Part model, mm, in its own coordinate system. Face numbers are marked on the shaded views. A direction names the side the tool comes from. Give positions to 0.01 mm unless a question says otherwise; leave off trailing zeros. Write each loop counter-clockwise with the first axis right and the second up, starting at its lowest first coordinate (ties: lowest second). Pieces come first, ordered by that corner, then holes. Notation, with made-up numbers: M -29,-24.5 L -13,-24.5 A17 cw -13,-13.5 Z; hole C 27.25,56.25 d9. An arc over 180 degrees is marked long. Use a Markdown table: item, result.
```python
from build123d import *

# Parameters (mm, degrees)
CROQUIS1_R              = 50
SALIENTE_EXTRUIR1_DEPTH = 40
CROQUIS2_R              = 45
CROQUIS2_R_2            = 32.5
CORTAR_EXTRUIR1_DEPTH   = 1.5
CROQUIS3_R              = 13
CROQUIS3_R_2            = 5
CORTAR_EXTRUIR2_DEPTH   = 8
CROQUIS4_R              = 5
CORTAR_EXTRUIR3_DEPTH   = 10


with BuildPart() as part:
    # Croquis1 → Saliente-Extruir1 (new body)
    with BuildSketch(Plane.XY):
        Circle(CROQUIS1_R)
    extrude(amount=SALIENTE_EXTRUIR1_DEPTH)

    # Croquis2 → Cortar-Extruir1 (cut)
    with BuildSketch(Plane(origin=(0, 0, 0), x_dir=(-1, 0, 0), z_dir=(0, 0, -1))):
        Circle(CROQUIS2_R)
        Circle(CROQUIS2_R_2, mode=Mode.SUBTRACT)
    extrude(amount=-CORTAR_EXTRUIR1_DEPTH, mode=Mode.SUBTRACT)

    # Croquis3 → Cortar-Extruir2 (cut)
    with BuildSketch(Plane(origin=(0, 0, 0), x_dir=(-1, 0, 0), z_dir=(0, 0, -1))):
        Circle(CROQUIS3_R)
        Circle(CROQUIS3_R_2, mode=Mode.SUBTRACT)
    extrude(amount=-CORTAR_EXTRUIR2_DEPTH, mode=Mode.SUBTRACT)

    # Croquis4 → Cortar-Extruir3 (cut)
    with BuildSketch(Plane(origin=(0, 0, 0), x_dir=(-1, 0, 0), z_dir=(0, 0, -1))):
        Circle(CROQUIS4_R)
    extrude(amount=-CORTAR_EXTRUIR3_DEPTH, mode=Mode.SUBTRACT)


solid = part.part
```
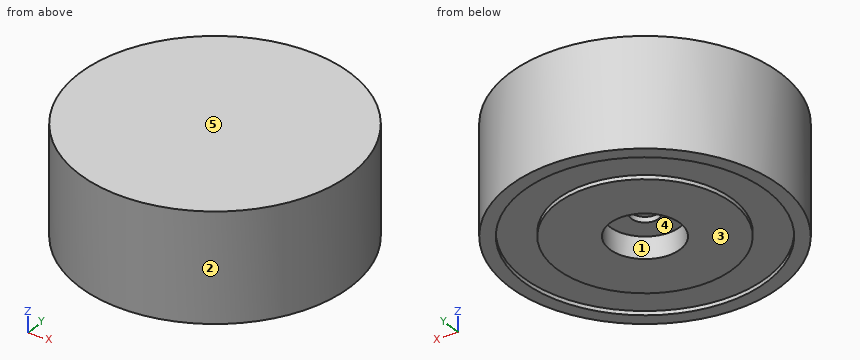
1. Drill centre lines: L1, parallel to Y at x = 0, z = 8.85; L2, parallel to Y at x = 0, z = 6; L3, parallel to Z at x = -14.5, y = -40.5. Where is each one in solid material? Low to high.
Findings below:
| item | result |
|---|---|
| L1 | -50 to -5, 5 to 50 |
| L2 | -50 to -13, 13 to 50 |
| L3 | 1.5 to 40 |
2. Cut at C-C, the plane z = 37.5. Give the cut face in (x, y), then the cut area to 3 significant figures.
Findings below:
| item | result |
|---|---|
| outline | C 0,0 d100 |
| area | 7,850 mm2 |
3. Drop flat-ended pins along their axis: P1, Ø10, axis at x = -32.5, z = 26, coming from the +Y side; P2, Ø8, axis at x = -1, y = -0.5, coming from the -Z side; P3, Ø3, axis at x = 1, z = 28.5, coming from the +Y side. Give the stop position or say it passes through.
Findings below:
| item | result |
|---|---|
| P1 | y = 41.76 |
| P2 | z = 8 |
| P3 | y = 50 |
4. Two-plate mould, pull along Y, no slides. Class the marked faces 1, 2 and 3: released by +Y, released by -Y, zero draft, split by the parting line, or undercut.
Findings below:
| item | result |
|---|---|
| face 1 | undercut |
| face 2 | split by the parting line |
| face 3 | zero draft |
5. Cut at D-D, the plane y = 38. Give the cut face in (x, z).
Findings below:
| item | result |
|---|---|
| outline | M -32.5,0 L -24.1,0 L -24.1,1.5 L 24.1,1.5 L 24.1,0 L 32.5,0 L 32.5,40 L -32.5,40 Z |
6. Tool access for the marked faces 4 and 5: list every direction of +Z, -Z, +X, -X, +Y, -Y with a clear straight run to the whole face (end or side of a thin tool).
Findings below:
| item | result |
|---|---|
| face 4 | -Z |
| face 5 | +Z, +X, -X, +Y, -Y |
7. Cut at A-A, the plane y = 0. Give the cut face in (x, z), then the cut area to 3 significant figures.
Findings below:
| item | result |
|---|---|
| outline | M -50,0 L -45,0 L -45,1.5 L -32.5,1.5 L -32.5,0 L -13,0 L -13,8 L -5,8 L -5,10 L 5,10 L 5,8 L 13,8 L 13,0 L 32.5,0 L 32.5,1.5 L 45,1.5 L 45,0 L 50,0 L 50,40 L -50,40 Z |
| area | 3,730 mm2 |
